```python
from build123d import *

# Parameters (mm, degrees)
SKETCH1_R           = 15.359074057
BOSS_EXTRUDE1_DEPTH = 50.8
BOSS_EXTRUDE2_DEPTH = 12.7
SKETCH3_R           = 6.35
BOSS_EXTRUDE3_DEPTH = 50.8


with BuildPart() as part:
    # Sketch1 → Boss-Extrude1 (new body)
    with BuildSketch(Plane.XY):
        Circle(SKETCH1_R)
    extrude(amount=BOSS_EXTRUDE1_DEPTH)

    # Sketch2 → Boss-Extrude2 (add)
    with BuildSketch(Plane(origin=(0, 0, 0), x_dir=(-1, 0, 0), z_dir=(0, 0, -1))):
        with BuildLine():
            Line((-31.75, 0), (-25.57013776, -31.75))
            ThreePointArc((-25.57013776, -31.75), (0, -52.822994947), (25.57013776, -31.75))
            Line((25.57013776, -31.75), (31.75, 0))
            ThreePointArc((31.75, 0), (0, 38.525699643), (-31.75, 0))
        make_face()
    extrude(amount=BOSS_EXTRUDE2_DEPTH)

    # Sketch3 → Boss-Extrude3 (add)
    with BuildSketch(Plane.XY):
        with Locations((0, -38.777693264)):
            Circle(SKETCH3_R)
    extrude(amount=BOSS_EXTRUDE3_DEPTH)


solid = part.part
```
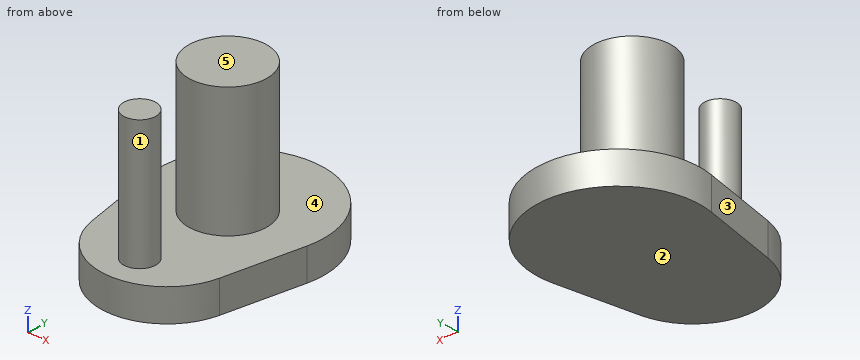
Part model, mm, in its own coordinate system. Face numbers are marked on the shaded views. A direction names the side the tool comes from. Round coordinates to 2 decimals unless told otherwise and drop trailing zeros. Write each loop counter-clockwise with the first axis right and the second up, starting at its lowest first coordinate (ties: lowest second). Pieces come first, ordered by that corner, then holes.
Item 1: Cut at C-C, the plane z = 44. Give the cut face in (x, y), plus the area to 3 significant figures.
Results:
outline: circle Ø30.72 at (0, 0); circle Ø12.7 at (0, -38.78)
area: 868 mm2
Item 2: Cut at B-B, the plane y = -42.5. Give the cut face in (x, z), plus the area to 3 significant figures.
Results:
outline: (-20.77, -12.7) - (20.77, -12.7) - (20.77, 0) - (5.14, 0) - (5.14, 50.8) - (-5.14, 50.8) - (-5.14, 0) - (-20.77, 0) - close
area: 1,050 mm2
Item 3: Probe L1, parallel to Z at x = -5, y = -32; L2, parallel to Y at x = 4, z = 21.5; L3, parallel to Y at x = 5, z = 20. List the from-to ranges inside material, lowest first.
Results:
L1: z = -12.7 to 0
L2: y = -43.71 to -33.85, -14.83 to 14.83
L3: y = -42.69 to -34.86, -14.52 to 14.52
Item 4: Drop flat-ended pins along their axis: pin 1 Ø4 at (x, z) = (-6.5, 35.5) entering from -Y; pin 2 Ø4 at (x, z) = (-13, 0.5) entering from +Y; pin 3 Ø3 at (y, z) = (4, 12) entering from -X; pin 4 Ø4 at (y, z) = (-28.5, 14) entering from -X. Give the stop position or say it passes through.
Results:
pin 1: stops at y = -43.26
pin 2: stops at y = 36.57
pin 3: stops at x = -15.15
pin 4: passes through
Item 5: Cut at A-A, the plane x = 0. Give the cut face in (y, z), plus the area to 3 significant figures.
Results:
outline: (-52.82, -12.7) - (38.53, -12.7) - (38.53, 0) - (15.36, 0) - (15.36, 50.8) - (-15.36, 50.8) - (-15.36, 0) - (-32.43, 0) - (-32.43, 50.8) - (-45.13, 50.8) - (-45.13, 0) - (-52.82, 0) - close
area: 3,370 mm2
Item 6: Which spindle directions (+Z, -Z, +X, -X, +Y, -Y) get a long thin tool onto all of the face, cutting with end or side? Do the marked faces 4 and 5. Say none if no direction does.
Results:
face 4: +Z
face 5: +Z, +X, -X, +Y, -Y
Item 7: Two-plate mould, pull along Y, no slides. Class the marked faces 1, 2 and 3: +Y half, -Y half, draft (parallel to the pull), parting line (faces both ways), or undercut.
Results:
face 1: undercut
face 2: draft
face 3: -Y half
Item 8: Cut at D-D, the plane y = -3. Give the cut face in (x, z).
Results:
outline: (-31.17, -12.7) - (31.17, -12.7) - (31.17, 0) - (15.06, 0) - (15.06, 50.8) - (-15.06, 50.8) - (-15.06, 0) - (-31.17, 0) - close
